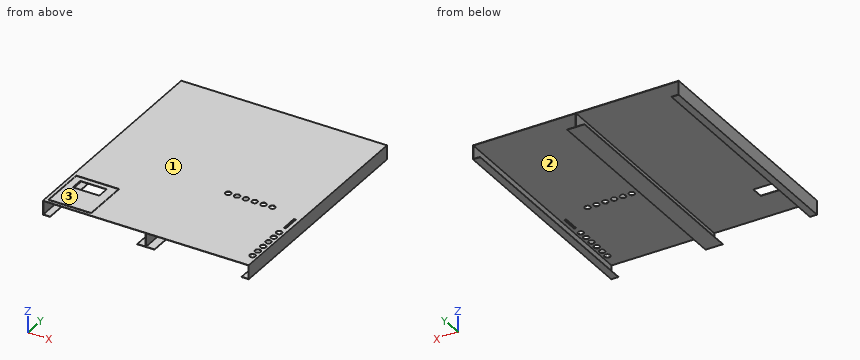
```python
from build123d import *

# Parameters (mm, degrees)
F1_DEPTH = 325
F3_D     = 16
F3_DEPTH = 5
F3_TIP   = 4.8068849522
F2_W     = 6
F2_H     = 13
F2_W_2   = 75
F2_H_2   = 35
F4_DEPTH = 25
F6_DEPTH = 1
F8_DEPTH = 325


# Not quite as in the source:
# - a feature names something its author has since deleted; it is built from what else it names


with BuildPart() as f1:
    # F0 (on Front) → F1 (new body, symmetric)
    with BuildSketch(Plane.XZ):
        Polygon((-291, 20), (-291, -20), (-271, -20), (-271, -19.1), (-290.1, -19.1), (-290.1, 19.1), (290.1, 19.1), (290.1, -19.1), (271, -19.1), (271, -20), (291, -20), (291, 20), align=None)
    extrude(amount=F1_DEPTH, both=True)

    # F3
    with Locations(Plane.XY.offset(20)):
        with Locations((276, -282), (276, -257), (276, -232), (276, -207), (276, -182), (201, -64.213295877), (176, -64.213295877), (151, -64.213295877), (126, -64.213295877), (101, -64.213295877), (76, -64.213295877), (276, -157)):
            Hole(F3_D / 2, depth=F3_DEPTH)
            with Locations((0, 0, -(F3_DEPTH + F3_TIP / 2))):  # 118° drill point
                Cone(0, F3_D / 2, F3_TIP, mode=Mode.SUBTRACT)

    # F2 (on face) → F4 (cut)
    with BuildSketch(Plane.XY.offset(20)):
        with Locations((277, -125.5)):
            Rectangle(F2_W, F2_H)
        with Locations((-223.5, -217.5)):
            Rectangle(F2_W_2, F2_H_2)
        with Locations((277, -108.5)):
            Rectangle(F2_W, F2_H)
        with Locations((277, -91.5)):
            Rectangle(F2_W, F2_H)
    extrude(amount=-F4_DEPTH, mode=Mode.SUBTRACT)

    # F5 (on face) → F6 (join)
    with BuildSketch(Plane.XY.offset(20)):
        with BuildLine():
            Line((-161.5, -184.5), (-280.5, -184.5))
            ThreePointArc((-280.5, -184.5), (-281.2071067812, -184.7928932188), (-281.5, -185.5))
            Line((-281.5, -185.5), (-281.5, -314.5))
            ThreePointArc((-281.5, -314.5), (-281.2071067812, -315.2071067812), (-280.5, -315.5))
            Line((-280.5, -315.5), (-161.5, -315.5))
            ThreePointArc((-161.5, -315.5), (-160.7928932188, -315.2071067812), (-160.5, -314.5))
            Line((-160.5, -314.5), (-160.5, -185.5))
            ThreePointArc((-160.5, -185.5), (-160.7928932188, -184.7928932188), (-161.5, -184.5))
        make_face()
        with BuildLine():
            ThreePointArc((-281, -186), (-280.7071067812, -185.2928932188), (-280, -185))
            Line((-280, -185), (-162, -185))
            ThreePointArc((-162, -185), (-161.2928932188, -185.2928932188), (-161, -186))
            Line((-161, -186), (-161, -314))
            ThreePointArc((-161, -314), (-161.2928932188, -314.7071067812), (-162, -315))
            Line((-162, -315), (-280, -315))
            ThreePointArc((-280, -315), (-280.7071067812, -314.7071067812), (-281, -314))
            Line((-281, -314), (-281, -186))
        make_face(mode=Mode.SUBTRACT)
    extrude(amount=F6_DEPTH)

    # F7 (on Front) → F8 (join, symmetric)
    with BuildSketch(Plane.XZ):
        Polygon((-24.3627466261, -20), (24.3627466261, -20), (24.3627466261, -19.1), (0.4681956061, -19.1), (0.4681956061, 20), (-0.4318043939, 20), (-0.4318043939, -19.1), (-24.3627466261, -19.1), align=None)
    extrude(amount=F8_DEPTH, both=True)


solid = f1.part
```
Design review of the part built by this model. Coordinates are the model's own, in mm. Face numbers are marked on the shaded views. Coordinates: 2 decimals unless noted, no trailing zeros. Loops run counter-clockwise (first coordinate to the right, second up) from the corner with the lowest first, then second, coordinate; pieces in that order, holes last.
Q1. We need section C-C on x = 101. State the section outline as (y, z) points.
Reported:
outline: (-325, 19.1) - (-72.21, 19.1) - (-72.21, 20) - (-325, 20) - close; (-56.21, 19.1) - (325, 19.1) - (325, 20) - (-56.21, 20) - close
Q2. We need section D-D on y = -207. State how many separate pieces and enclosed holes the cut face has, and give its area (3 significant figures).
Reported:
separate pieces: 3
enclosed holes: 0
area: 626 mm2
Q3. The part is to be moulded in two halves that separate along X. For the marked faces 1, 2 and 3, say which applies: +X half, -X half, draft (parallel to the pull), parting line (faces both ways), or undercut.
Reported:
face 1: draft
face 2: undercut
face 3: undercut
Q4. For pin 1 (5 mm diameter, centred on x = -50, y = 253, fed in from -Z); pin 2 (15.5 mm diameter, centred on x = -281.5, y = -39, fed in from +Z); pin 3 (0.8 mm diameter, centred on x = -202, z = 20.5, fed in from -Y); pin 4 (5 mm diameter, centred on x = 1.5, z = 3, fed in from +Y), all flat-tipped, find the tip position at first contact; note any pin that passes through.
Reported:
pin 1: stops at z = 19.1
pin 2: stops at z = 20
pin 3: stops at y = -315.5
pin 4: stops at y = 325
Q5. We need section A-A on z = 3. State the section outline as (x, y) points, and give its area (4 significant figures).
Reported:
outline: (-291, -325) - (-290.1, -325) - (-290.1, 325) - (-291, 325) - close; (-0.43, -325) - (0.47, -325) - (0.47, 325) - (-0.43, 325) - close; (290.1, -325) - (291, -325) - (291, 325) - (290.1, 325) - close
area: 1,755 mm2
Q6. To check wall thickness, follow line 1 (X direction, y = 66, z = -11.5); line 2 (Y direction, x = 101, z = 19.8); line 3 (Z direction, x = -136, y = 133). State the ranges of each line that lie inside material, in increasing order.
Reported:
line 1: x = -291 to -290.1, -0.43 to 0.47, 290.1 to 291
line 2: y = -325 to -72.21, -56.21 to 325
line 3: z = 19.1 to 20
